Input: part model. Units: mm. Frame: model coordinates. Face numbers are marked on the shaded views. A direction names the side the tool comes from. Coordinates: 2 decimals unless noted, no trailing zeros. One line per question, with ' | ' between items.
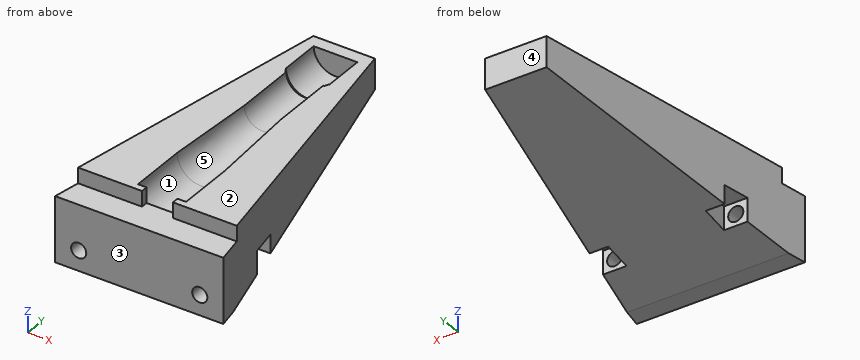
```python
from build123d import *

# Parameters (mm, degrees)
SKETCH_2_W               = 50
SKETCH_2_H               = 50
EXTRUDE_1_DEPTH          = 90
EXTRUDE_1_TAPER          = 10
SKETCH_3_W               = 215.720321278
SKETCH_3_H               = 290.879799434
CUT_EXTRUDE_1_DEPTH      = 97.695398174
SKETCH_7_W               = 4.6
SKETCH_7_H               = 23.792731937
SKETCH_8_W               = 50
SKETCH_8_H               = 4.6
CUT_EXTRUDE_2_DEPTH      = 8
SKETCH_9_W               = 9.2
SKETCH_9_H               = 9.2
CUT_EXTRUDE_3_DEPTH      = 4.6
SKETCH_10_W              = 7
SKETCH_10_H              = 8
CUT_EXTRUDE_4_DEPTH      = 10.5
SKETCH_11_R              = 2.25
CUT_EXTRUDE_5_DEPTH      = 20
CUT_EXTRUDE_6_DEPTH      = 97.695398174
CUT_EXTRUDE_6_DEPTH_BACK = 97.695398174
SKETCH_12_W              = 75.055418853
SKETCH_12_H              = 23.361905794


with BuildPart() as part:
    # 草圖2 → 填料-伸長1 (new body)
    with BuildSketch(Plane(origin=(0, 0, 0), x_dir=(1, 0, 0), z_dir=(0, 1, 0))):
        Rectangle(SKETCH_2_W, SKETCH_2_H)
    extrude(amount=EXTRUDE_1_DEPTH, taper=EXTRUDE_1_TAPER)

    # 草圖3 → 除料-伸長1 (cut, through all)
    with BuildSketch(Plane.XY):
        Rectangle(SKETCH_3_W, SKETCH_3_H)
    extrude(amount=CUT_EXTRUDE_1_DEPTH, mode=Mode.SUBTRACT)


with BuildPart() as body_2:
    # stick_antenna_434MHz: read off the stored shape, not the designer's step
    # stick_antenna_434MHz outline → stick_antenna_434MHz (revolve)
    with BuildSketch(Plane.XY):
        Polygon((0, 86.2), (0, 10), (6.65, 10), (6.65, 27.2), (5, 54.2), (5, 73.2), (5.5, 73.2), (6, 74.2), (6, 86.2), align=None)
    revolve(axis=Axis((0, 0, 0), (0, 1, 0)))


with BuildPart() as part_1:
    add(part.part)

    # Other 1: read off the stored shape, not the designer's step
    # Other 1: cut body 2
    add(body_2.part, mode=Mode.SUBTRACT)

    # 草圖14 → 除料-旋轉2 (revolve, cut)
    with BuildSketch(Plane.XY):
        Polygon((7.15, 10), (0, 10), (0, 86.2), (6.5, 86.2), (6.5, 74.081966011), (5.809016994, 72.7), (5.5, 72.7), (5.5, 54.21526354), (7.15, 27.21526354), align=None)
    revolve(axis=Axis((0, 88.093709872, 0), (0, -1, 0)), mode=Mode.SUBTRACT)

    # 草圖7 → 除料-旋轉1 (revolve, cut)
    with BuildSketch(Plane.XY):
        with Locations((2.3, 11.896365969)):
            Rectangle(SKETCH_7_W, SKETCH_7_H)
    revolve(axis=Axis((0, 30.263839144, 0), (0, -1, 0)), mode=Mode.SUBTRACT)

    # 草圖8 → 除料-伸長2 (cut)
    with BuildSketch(Plane.XZ):
        with Locations((0, -2.3)):
            Rectangle(SKETCH_8_W, SKETCH_8_H)
    extrude(amount=-CUT_EXTRUDE_2_DEPTH, mode=Mode.SUBTRACT)

    # 草圖9 → 除料-伸長3 (cut)
    with BuildSketch(Plane.XY):
        with Locations((0, 5.4)):
            Rectangle(SKETCH_9_W, SKETCH_9_H)
    extrude(amount=-CUT_EXTRUDE_3_DEPTH, mode=Mode.SUBTRACT)

    # 草圖10 → 除料-伸長4 (cut)
    with BuildSketch(Plane.XY.offset(-25)):
        with Locations((-18, 24)):
            Rectangle(SKETCH_10_W, SKETCH_10_H)
    cut_extrude_4 = extrude(amount=CUT_EXTRUDE_4_DEPTH, mode=Mode.SUBTRACT)

    # 草圖11 → 除料-伸長5 (cut)
    with BuildSketch(Plane.XZ):
        with Locations(Location((-18, -18, 0), (0, 0, 270))):
            Circle(SKETCH_11_R)
        with Locations(Location((18, -18, 0), (0, 0, 90))):
            Circle(SKETCH_11_R)
    extrude(amount=-CUT_EXTRUDE_5_DEPTH, mode=Mode.SUBTRACT)

    # 鏡射2: 除料-伸長4 across plane
    add(cut_extrude_4.mirror(Plane(origin=(0, 0, 0), x_dir=(0, 0, 1), z_dir=(1, 0, 0))), mode=Mode.SUBTRACT)

    # 草圖12 → 除料-伸長6 (cut, two sides: drawn at the far end of the back side and taken through both)
    with BuildSketch(Plane(origin=(0, 0, 0), x_dir=(0, 0, -1), z_dir=(1, 0, 0)).offset(-CUT_EXTRUDE_6_DEPTH_BACK)):
        with Locations((61.527709427, 0)):
            Rectangle(SKETCH_12_W, SKETCH_12_H)
    extrude(amount=CUT_EXTRUDE_6_DEPTH + CUT_EXTRUDE_6_DEPTH_BACK, mode=Mode.SUBTRACT)


solid = part_1.part
```
1. Pin query (flat end, axial travel): pin 1 Ø6 at (x, y) = (1, 81) entering from -Z; pin 2 Ø5.5 at (x, y) = (-17, 23) entering from -Z; pin 3 Ø0.6 at (y, z) = (9.5, -3.5) entering from -X. Return the tip coordinate at first contact, or that it passes through.
Recorded:
pin 1: stops at z = -11.25 | pin 2: stops at z = -21.15 | pin 3: stops at x = -23.38
2. Access query for the marked faces 4 and 5. Directions: +Z, -Z, +X, -X, +Y, -Y. A direction counts if a zero-diameter tool reaches every point of the face in a straight line with its end or side. Return the directions, or none.
Recorded:
face 4: +Z, -Z, +X, -X, +Y | face 5: +Z
3. Cut plane A-A, the plane z = -18. State how many separate pieces and enclosed holes the cut face has, and give its area (3 significant figures).
Recorded:
separate pieces: 3 | enclosed holes: 0 | area: 1,430 mm^2
4. Ray query, line 1 (X direction, y = 11.75, z = -18); line 2 (Z direction, x = 18, y = 4); line 3 (Z direction, x = -17, y = 26). Return the intervals inside material, ascending. Write a range as [from, to].
Recorded:
line 1: x = [-22.93, -20.25], [-15.75, 15.75], [20.25, 22.93] | line 2: z = [-24, -20.25], [-15.75, -4.6] | line 3: z = [-14.5, 0]
5. Mould query, pull axis Y, two halves, no side actions, for the marked faces 1, 2 and 3. Classes: released by +Y, released by -Y, zero draft, split by the parting line, or undercut.
Recorded:
face 1: undercut | face 2: zero draft | face 3: released by -Y
